Check sheet for the modelled part. Datum: model origin and axes. Units: mm. Face numbers are marked on the shaded views. A direction names the side the tool comes from. Coordinates: 2 decimals unless noted, no trailing zeros. Write each loop counter-clockwise with the first axis right and the second up, starting at its lowest first coordinate (ties: lowest second). Pieces come first, ordered by that corner, then holes. Notation, with made-up numbers: M -22.75,-22 L 31.25,-22 A24 cw 31.25,4 Z; hole C 81,48.25 d7. An arc over 180 degrees is marked long. Answer as CSV lines item,"result". Start each with the question number.
Q1. Sectioned sample at D-D, the plane y = 2.6. Record the cut outline in (x, z).
Q2. Sectioned sample at A-A, the plane z = 0. Record the cut outline in (x, y).
Q3. Mould release check, pull along X, two halves, no side actions. Record for the marked faces 1, 2, 3 and 4: pulls with the +X half, pulls with the -X half, needs draft (parallel to the pull), parting line crosses it, or undercut.
Q4. Access from +Z, -Z, +X, -X, +Y, -Y to the whole of each face (thin tool, end or side, straight path). Record for the marked faces 5, 6 and 7.
Q5. Sectioned sample at B-B, the plane y = 1.7. Record the cut outline in (x, z).
Q6. Depth check by flat-ended pin: pin 1 Ø1.5 at (x, y) = (2, 2) entering from +Z; pin 2 Ø1.1 at (x, z) = (-0.5, 0) entering from +Y. Enter the tip coordinate at first touch or a pass-through.
Q7. Thickness scan on line 1 along X through (y, z) = (2.1, 0); line 2 along X through (y, z) = (3.4, 0); line 3 along Y through (x, z) = (0.1, 1.6). Record the ranges inside material, lowest first. Write a range as from..to.
Q8. Sectioned sample at C-C, the plane y = 3. Record the cut outline in (x, z).
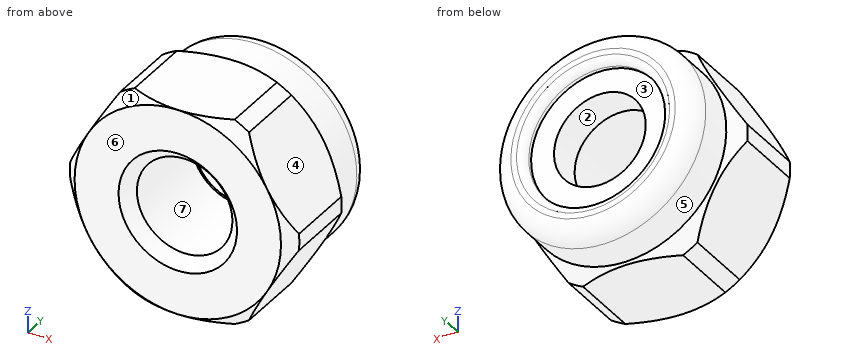
from build123d import *

# Parameters (mm, degrees)
SKETCH3_OUTSIDE_W     = 9.868
SKETCH3_OUTSIDE_H     = 9.868
CUT_EXTRUDE1_DEPTH    = 10
FILLET2_R             = 0.5
FILLET3_R             = 0.2
M3_TAPPED_HOLE4_D     = 2.5
M3_TAPPED_HOLE4_DEPTH = 21.5
M3_TAPPED_HOLE4_TIP   = 0.751075774
CHAMFER1_SIZE         = 0.3
SKETCH6_W             = 0.6
SKETCH6_H             = 0.9


with BuildPart() as part:
    # Sketch1 → Revolve1 (revolve)
    with BuildSketch(Plane.XY, mode=Mode.PRIVATE) as revolve1_sk:
        Polygon((1, 0), (2.7, 0), (3, 0.3), (3, 2.15), (2.65, 2.5), (2.65, 3.9), (1.8, 3.9), (1.8, 2.7), (1, 2.7), align=None)
    revolve(revolve1_sk.sketch.rotate(Axis((0, 0, 0), (0, 1, 0)), 90), axis=Axis((0, 0, 0), (0, 1, 0)))

    # Sketch3 outside → Cut-Extrude1 (cut)
    with BuildSketch(Plane(origin=(0, 3.9, 0), x_dir=(1, 0, 0), z_dir=(0, 1, 0))):
        Rectangle(SKETCH3_OUTSIDE_W, SKETCH3_OUTSIDE_H)
        Polygon((3.117691454, 0), (1.558845727, 2.7), (-1.558845727, 2.7), (-3.117691454, 0), (-1.558845727, -2.7), (1.558845727, -2.7), align=None, mode=Mode.SUBTRACT)
    extrude(amount=-CUT_EXTRUDE1_DEPTH, mode=Mode.SUBTRACT)

    # Fillet2
    fillet2_edges = [part.edges().sort_by_distance(p)[0] for p in [
        (0, 3.9, 2.65),
    ]]
    fillet(fillet2_edges, radius=FILLET2_R)

    # Fillet3
    fillet3_edges = [part.edges().sort_by_distance(p)[0] for p in [
        (0, 3.9, 1.8),
    ]]
    fillet(fillet3_edges, radius=FILLET3_R)

    # M3 Tapped Hole4
    with Locations(Plane(origin=(0, 0, 0), x_dir=(0, 0, -1), z_dir=(0, -1, 0))):
        with Locations((0, 0)):
            Hole(M3_TAPPED_HOLE4_D / 2, depth=M3_TAPPED_HOLE4_DEPTH)
            with Locations((0, 0, -(M3_TAPPED_HOLE4_DEPTH + M3_TAPPED_HOLE4_TIP / 2))):  # 118° drill point
                Cone(0, M3_TAPPED_HOLE4_D / 2, M3_TAPPED_HOLE4_TIP, mode=Mode.SUBTRACT)

    # Chamfer1
    chamfer1_edges = [part.edges().sort_by_distance(p)[0] for p in [
        (0, 0, -1.25),
    ]]
    chamfer(chamfer1_edges, length=CHAMFER1_SIZE)

    # Sketch6 → Revolve2 (revolve)
    with BuildSketch(Plane.XY, mode=Mode.PRIVATE) as revolve2_sk:
        with Locations((-1.5, 3.15)):
            Rectangle(SKETCH6_W, SKETCH6_H)
    revolve(revolve2_sk.sketch.rotate(Axis((0, 0, 0), (0, 1, 0)), 270), axis=Axis((0, 0, 0), (0, 1, 0)))


solid = part.part
Output:
1,outline,"C 0,0 d5.3; hole C 0,0 d2.5"
2,outline,"M -3,0.3 L -2.7,0 L -1.55,0 L -1.25,0.3 L -1.25,2.7 L -1.2,2.7 L -1.2,3.6 L -1.8,3.6 L -1.8,3.7 A0.2 ccw -2,3.9 L -2.15,3.9 A0.5 ccw -2.65,3.4 L -2.65,2.5 L -3,2.15 Z; M 1.2,2.7 L 1.25,2.7 L 1.25,0.3 L 1.55,0 L 2.7,0 L 3,0.3 L 3,2.15 L 2.65,2.5 L 2.65,3.4 A0.5 ccw 2.15,3.9 L 2,3.9 A0.2 ccw 1.8,3.7 L 1.8,3.6 L 1.2,3.6 Z"
3,face 1,"pulls with the -X half"
3,face 2,"undercut"
3,face 3,"undercut"
3,face 4,"pulls with the +X half"
4,face 5,"+Y"
4,face 6,"+Z, -Z, +X, -X, -Y"
4,face 7,"-Y"
5,outline,"M -2.99,-0.22 L -1.68,-2.48 A3 ccw -1.31,-2.7 L 1.31,-2.7 A3 ccw 1.68,-2.48 L 2.99,-0.22 A3 ccw 2.99,0.22 L 1.68,2.48 A3 ccw 1.31,2.7 L -1.31,2.7 A3 ccw -1.68,2.48 L -2.99,0.22 A3 ccw Z; hole C 0,0 d2.5"
6,pin 1,"stops at z = 2.7"
6,pin 2,"passes through"
7,line 1,"x = -3..-1.25, 1.25..3"
7,line 2,"x = -2.65..-1.2, 1.2..2.65"
7,line 3,"y = 0..3.6"
8,outline,"C 0,0 d5.3; hole C 0,0 d2.4"
